Verification items for the finished model (mm, model axes). Face numbers are marked on the shaded views. Give positions to 0.01 mm unless a question says otherwise; leave off trailing zeros. Order: outer loops, then holes, each group sorted by start corner. A loop starts at its lowest first (then second) coordinate and runs counter-clockwise, first axis right, second up. Notation, with made-up numbers: (87, -25) - (94, -25) arc R8 cw to (94, -10) - close; hole circle Ø8 at (11, 37.5). An arc over 180 degrees is marked (long way). Answer as a JSON object with one key per item and string values.
```python
from build123d import *

# Parameters (mm, degrees)
F2_R = 8
F3_R = 8


with BuildPart() as f1:
    # F0 (on Front) → F1 (revolve)
    with BuildSketch(Plane.XZ):
        Polygon((5.534274, 53.437501), (0, 53.437501), (0, 0), (8.074597, 0), (9.715894, 3.241377), (9.715894, 7.051861), (8.074597, 11.043796), (8.074597, 27.870369), (6.268315, 29.188959), (8.074597, 31.66331), (9.526211, 37.46976), (8.074597, 42.550407), (3.901211, 49.264114), (5.534274, 49.98992), align=None)
    revolve(axis=Axis((0, 0, 26.718751), (0, 0, 1)))

    # F2
    f2_edges = [f1.edges().sort_by_distance(p)[0] for p in [
        (-8.074597, 0, 42.550407),
        (-9.526211, 0, 37.46976),
        (-8.074597, 0, 31.66331),
    ]]
    fillet(f2_edges, radius=F2_R)

    # F3
    f3_edges = [f1.edges().sort_by_distance(p)[0] for p in [
        (-8.074597, 0, 11.043796),
        (-9.715894, 0, 7.051861),
        (-9.715894, 0, 3.241377),
    ]]
    fillet(f3_edges, radius=F3_R)


solid = f1.part
```
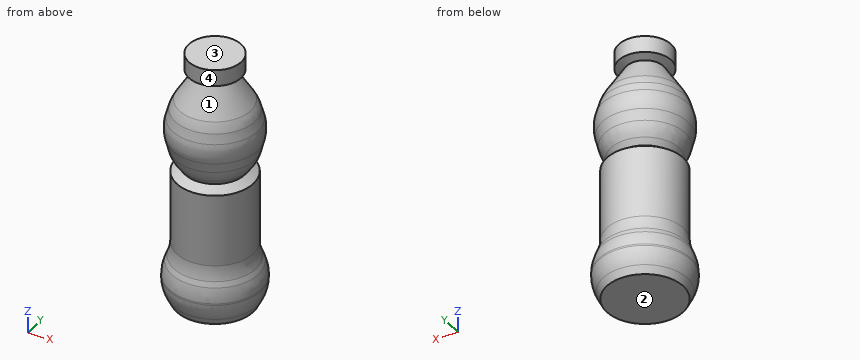
(1) Material ranges on line 1 along X through (y, z) = (3.75, 16.5); line 2 along Z through (x, y) = (5, -6); line 3 along Z through (x, y) = (-3.75, 2), recorded low to high. Write a range as [from, to].
Computed values:
{"line 1": "x = [-7.15, 7.15]", "line 2": "z = [0, 28.06], [31.47, 42.92]", "line 3": "z = [0, 48.7], [49.42, 53.44]"}
(2) Gauge pin test, flat ends, axial feed: pin 1 Ø1 at (x, z) = (-3.5, 33.5) entering from +Y; pin 2 Ø8 at (x, z) = (-3, 34.5) entering from -Y; pin 3 Ø8 at (y, z) = (-7, 37) entering from -X. Record the tip position at first contact, or that the pin passes through.
Computed values:
{"pin 1": "stops at y = 8.03", "pin 2": "stops at y = -9.24", "pin 3": "stops at x = -8.74"}
(3) Release check for a two-part mould opening along Z. For the marked faces 1, 2, 3 and 4 record: pulls with the +Z half, pulls with the -Z half, needs draft (parallel to the pull), parting line crosses it, or undercut.
Computed values:
{"face 1": "undercut", "face 2": "pulls with the -Z half", "face 3": "pulls with the +Z half", "face 4": "needs draft"}
(4) Section check A-A (z = 18). Record the cut outline in (x, y), then the cut area to 3 significant figures.
Computed values:
{"outline": "circle Ø16.15 at (0, 0)", "area": "205 mm²"}
